Geometry check sheet. Reference: the model listing, model coordinates, mm. Face numbers are marked on the shaded views. Give positions to 0.01 mm unless a question says otherwise; leave off trailing zeros. Write each loop counter-clockwise with the first axis right and the second up, starting at its lowest first coordinate (ties: lowest second). Pieces come first, ordered by that corner, then holes.
(1) Cross-section at B-B (z = -20). Record the boundary of the cut face in (x, y).
(2) Thickness scan on line 1 along X through (y, z) = (5.25, 53); line 2 along Z through (x, y) = (-7.25, 9); line 3 along Y through (x, z) = (-10, -13.5). Record the ranges inside material, lowest first.
(3) Cross-section at A-A (y = 0). Record the boundary of the cut face in (x, z).
(4) Depth check by flat-ended pin: P1, Ø15, axis at x = 4.5, z = 8.5, coming from the +Y side; P2, Ø15, axis at x = -2.5, z = 4, coming from the -Y side. Enter the tip coordinate at first touch or a pass-through.
(5) Cross-section at C-C (x = 7.5). Count the separate pieces of the cut face and the enclosed holes in it, and give its area (3 significant figures).
(6) Mould release check, pull along Z, two halves, no side actions. Record for the marked faces 1, 2, 3 and 4: +Z half, -Z half, draft (parallel to the pull), parting line (faces both ways), or undercut.
(7) Cross-section at D-D (z = 53). Record the boundary of the cut face in (x, y).
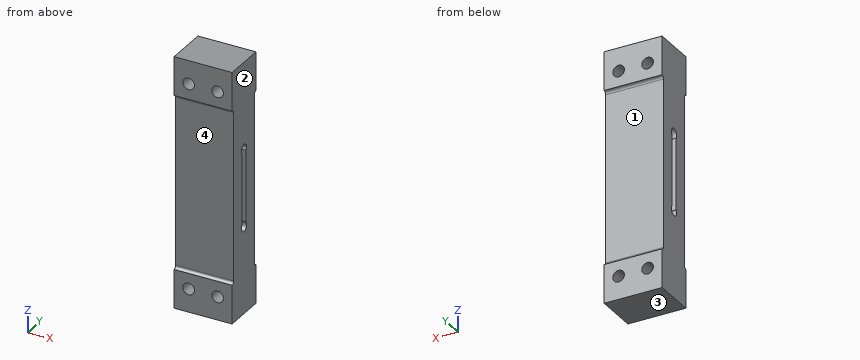
```python
from build123d import *

# Parameters (mm, degrees)
SKETCH1_W           = 130
SKETCH1_H           = 22
BOSS_EXTRUDE1_DEPTH = 15
SKETCH2_R           = 3
CUT_EXTRUDE1_DEPTH  = 71.242437315
SKETCH3_W           = 90
SKETCH3_H           = 1.5
CUT_EXTRUDE2_DEPTH  = 30
FILLET1_R           = 1.5


with BuildPart() as part:
    # Sketch1 → Boss-Extrude1 (new, symmetric)
    with BuildSketch(Plane(origin=(0, 0, 0), x_dir=(0, 0, -1), z_dir=(1, 0, 0))):
        Rectangle(SKETCH1_W, SKETCH1_H)
        with BuildLine():
            Line((-18.5, 2), (18.5, 2))
            ThreePointArc((18.5, 2), (22.5, 0), (18.5, -2))
            Line((18.5, -2), (-18.5, -2))
            ThreePointArc((-18.5, -2), (-22.5, 0), (-18.5, 2))
        make_face(mode=Mode.SUBTRACT)
    extrude(amount=BOSS_EXTRUDE1_DEPTH, both=True)

    # Sketch2 → Cut-Extrude1 (cut, through all)
    with BuildSketch(Plane(origin=(0, 11, 0), x_dir=(1, 0, 0), z_dir=(0, 1, 0))):
        with Locations(Location((-7.5, 53, 0), (0, 0, 270))):
            Circle(SKETCH2_R)
        with Locations(Location((7.5, 53, 0), (0, 0, 270))):
            Circle(SKETCH2_R)
        with Locations(Location((-7.5, -53, 0), (0, 0, 270))):
            Circle(SKETCH2_R)
        with Locations(Location((7.5, -53, 0), (0, 0, 270))):
            Circle(SKETCH2_R)
    extrude(amount=-CUT_EXTRUDE1_DEPTH, mode=Mode.SUBTRACT)

    # Sketch3 → Cut-Extrude2 (cut)
    with BuildSketch(Plane(origin=(15, 0, 0), x_dir=(0, 0, -1), z_dir=(1, 0, 0))):
        with Locations((0, -10.25)):
            Rectangle(SKETCH3_W, SKETCH3_H)
        with Locations((0, 10.25)):
            Rectangle(SKETCH3_W, SKETCH3_H)
    extrude(amount=-CUT_EXTRUDE2_DEPTH, mode=Mode.SUBTRACT)

    # Fillet1
    fillet1_edges = [part.edges().sort_by_distance(p)[0] for p in [
        (0, -9.5, 45),
        (0, -9.5, -45),
        (0, 9.5, -45),
        (0, 9.5, 45),
    ]]
    fillet(fillet1_edges, radius=FILLET1_R - 0.0001)  # a hair under: the kernel refuses the full size


solid = part.part
```
Reply:
1. outline: (-15, -9.5) - (15, -9.5) - (15, -2.5) - (-15, -2.5) - close; (-15, 2.5) - (15, 2.5) - (15, 9.5) - (-15, 9.5) - close
2. line 1: x = -15 to -10.5, -4.5 to 4.5, 10.5 to 15
2. line 2: z = -65 to -55.99, -50.01 to 50.01, 55.99 to 65
2. line 3: y = -9.5 to -2, 2 to 9.5
3. outline: (-15, -65) - (15, -65) - (15, -22.5) - (-15, -22.5) - close; (-15, 22.5) - (15, 22.5) - (15, 65) - (-15, 65) - close; hole circle Ø6 at (-7.5, -53); hole circle Ø6 at (-7.5, 53); hole circle Ø6 at (7.5, -53); hole circle Ø6 at (7.5, 53)
4. P1: stops at y = 9.5
4. P2: stops at y = -9.5
5. separate pieces: 3
5. enclosed holes: 1
5. area: 2,150 mm2
6. face 1: undercut
6. face 2: draft
6. face 3: -Z half
6. face 4: undercut
7. outline: (-15, -11) - (-10.5, -11) - (-10.5, 11) - (-15, 11) - close; (-4.5, -11) - (4.5, -11) - (4.5, 11) - (-4.5, 11) - close; (10.5, -11) - (15, -11) - (15, 11) - (10.5, 11) - close
